from build123d import *

# Parameters (mm, degrees)
SKETCH1_W                    = 25.4
SKETCH1_H                    = 21.844
BOLT_SIZE_WIDTH_HEIGHT_DEPTH = 7.62
FRONT_CURVE_DEPTH            = 22.844
SKETCH3_W                    = 25.4
SKETCH3_H                    = 21.844
REAR_CAP_DEPTH               = 1.27
WINGS_DEPTH                  = 21.844
HOOK_DEPTH_DEPTH             = 5.08
HOOK_HEIGHT_DEPTH            = 3.81
NUT_FLANGE_CLEARANCE_R       = 1.27
DECORATION_SIZE              = 2.54
CUT_EXTRUDE1_DEPTH           = 27.9240001


with BuildPart() as part:
    # Sketch1 → Bolt Size, Width, &Height (new body)
    with BuildSketch(Plane.XY):
        Rectangle(SKETCH1_W, SKETCH1_H)
        Polygon((0, 5.842), (-5.059320409, 2.921), (-5.059320409, -2.921), (0, -5.842), (5.059320409, -2.921), (5.059320409, 2.921), align=None, mode=Mode.SUBTRACT)
    extrude(amount=BOLT_SIZE_WIDTH_HEIGHT_DEPTH)

    # Sketch2 → Front Curve (cut, through all)
    with BuildSketch(Plane(origin=(0, 10.922, 0), x_dir=(1, 0, 0), z_dir=(0, 1, 0))):
        with BuildLine():
            Line((12.7, -7.62), (12.7, -3.81))
            ThreePointArc((12.7, -3.81), (0, -4.668549118), (-12.7, -3.81))
            Line((-12.7, -3.81), (-12.7, -7.62))
            Line((-12.7, -7.62), (12.7, -7.62))
        make_face()
    extrude(amount=-FRONT_CURVE_DEPTH, mode=Mode.SUBTRACT)

    # Sketch3 → Rear Cap (add)
    with BuildSketch(Plane(origin=(0, 0, 0), x_dir=(-1, 0, 0), z_dir=(0, 0, -1))):
        Rectangle(SKETCH3_W, SKETCH3_H)
        Polygon((-3.789320409, 2.187765158), (-3.789320409, -2.187765158), (0, -4.375530316), (3.789320409, -2.187765158), (3.789320409, 2.187765158), (0, 4.375530316), align=None, mode=Mode.SUBTRACT)
    extrude(amount=REAR_CAP_DEPTH)

    # Sketch6 → Wings (add)
    with BuildSketch(Plane.XZ.offset(10.922)):
        with BuildLine():
            ThreePointArc((-12.7, 3.81), (-26.59057897, 0.844499757), (-39.878681796, -4.17234179))
            Line((-39.878681796, -4.17234179), (-37.752420533, -8.732123784))
            ThreePointArc((-37.752420533, -8.732123784), (-25.500637389, -4.079733878), (-12.7, -1.27))
            Line((-12.7, -1.27), (-12.7, 3.81))
        make_face()
        with BuildLine():
            ThreePointArc((39.878681796, -4.17234179), (26.59057897, 0.844499757), (12.7, 3.81))
            Line((12.7, 3.81), (12.7, -1.27))
            ThreePointArc((12.7, -1.27), (25.500637389, -4.079733878), (37.752420533, -8.732123784))
            Line((37.752420533, -8.732123784), (39.878681796, -4.17234179))
        make_face()
    extrude(amount=-WINGS_DEPTH)

    # Sketch7 → Hook Depth (add)
    with BuildSketch(Plane(origin=(0, 10.922, 0), x_dir=(1, 0, 0), z_dir=(0, 1, 0))):
        with BuildLine():
            Line((12.7, 1.27), (-12.7, 1.27))
            ThreePointArc((-12.7, 1.27), (-25.500637389, 4.079733878), (-37.752420533, 8.732123784))
            Line((-37.752420533, 8.732123784), (-42.90498238, -2.317580756))
            ThreePointArc((-42.90498238, -2.317580756), (-31.916762044, -6.681838924), (-20.495660276, -9.738989543))
            Line((-20.495660276, -9.738989543), (-19.05, -2.725598334))
            ThreePointArc((-19.05, -2.725598334), (0, -4.668549118), (19.05, -2.725598334))
            Line((19.05, -2.725598334), (20.495660276, -9.738989543))
            ThreePointArc((20.495660276, -9.738989543), (31.916762044, -6.681838924), (42.90498238, -2.317580756))
            Line((42.90498238, -2.317580756), (37.752420533, 8.732123784))
            ThreePointArc((37.752420533, 8.732123784), (25.500637389, 4.079733878), (12.7, 1.27))
        make_face()
    extrude(amount=HOOK_DEPTH_DEPTH)

    # Sketch8 → Hook Height (add)
    with BuildSketch(Plane.XZ.offset(-10.922)):
        with BuildLine():
            ThreePointArc((-20.495660276, 9.738989543), (-31.916762044, 6.681838924), (-42.90498238, 2.317580756))
            Line((-42.90498238, 2.317580756), (-41.831531995, 0.015558977))
            ThreePointArc((-41.831531995, 0.015558977), (-31.118228667, 4.270626689), (-19.982874273, 7.251289698))
            Line((-19.982874273, 7.251289698), (-20.495660276, 9.738989543))
        make_face()
        with BuildLine():
            Line((41.831531995, 0.015558977), (42.90498238, 2.317580756))
            ThreePointArc((42.90498238, 2.317580756), (31.916762044, 6.681838924), (20.495660276, 9.738989543))
            Line((20.495660276, 9.738989543), (19.982874273, 7.251289698))
            ThreePointArc((19.982874273, 7.251289698), (31.118228667, 4.270626689), (41.831531995, 0.015558977))
        make_face()
    extrude(amount=HOOK_HEIGHT_DEPTH)

    # Nut Flange Clearance
    nut_flange_clearance_edges = [part.edges().sort_by_distance(p)[0] for p in [
        (5.059320409, 0, 4.532819603),
        (2.530342979, 4.3811058, 4.634616736),
        (-2.530342979, 4.3811058, 4.634616736),
        (-5.059320409, 0, 4.532819603),
        (-2.530342979, -4.3811058, 4.634616736),
        (2.530342979, -4.3811058, 4.634616736),
    ]]
    fillet(nut_flange_clearance_edges, radius=NUT_FLANGE_CLEARANCE_R)

    # Decoration
    decoration_edges = [part.edges().sort_by_distance(p)[0] for p in [
        (-42.368257188, 7.112, 1.166569866),
        (-20.239267274, 7.112, 8.49513962),
        (42.368257188, 7.112, 1.166569866),
        (20.239267274, 7.112, 8.49513962),
    ]]
    chamfer(decoration_edges, length=DECORATION_SIZE)

    # Sketch9 → Cut-Extrude1 (cut, through all)
    with BuildSketch(Plane(origin=(0, 16.002, 0), x_dir=(1, 0, 0), z_dir=(0, 1, 0))):
        with BuildLine():
            Line((42.90498238, -2.317580756), (39.878681796, 4.17234179))
            ThreePointArc((39.878681796, 4.17234179), (0, -4.668549118), (-39.878681796, 4.17234179))
            Line((-39.878681796, 4.17234179), (-42.90498238, -2.317580756))
            ThreePointArc((-42.90498238, -2.317580756), (0, -11.82938635), (42.90498238, -2.317580756))
        make_face()
    extrude(amount=-CUT_EXTRUDE1_DEPTH, mode=Mode.SUBTRACT)


solid = part.part
Here's how the part is built. I have some questions about the finished solid (model axes, mm). A direction names the side the tool comes from. Coordinates: 2 decimals unless noted, no trailing zeros. Loops run counter-clockwise (first coordinate to the right, second up) from the corner with the lowest first, then second, coordinate; pieces in that order, holes last. Notation, with made-up numbers: (-39, -13.5) -> (6, -13.5) arc R15 cw to (6, 2.5) -> close; hole circle Ø1 at (48, 38.25). An arc over 180 degrees is marked (long way). Use one line per item in the form item = value. Start each with the question number.
(1) Will these pins go through, and if not, where does the flat tip stop? pin 1 (3 mm diameter, centred on x = -6.5, y = -7, fed in from +Z); pin 2 (12.5 mm diameter, centred on x = -5, y = 5, fed in from -Z); pin 3 (8 mm diameter, centred on x = 1.5, y = -2, fed in from +Z).
(2) If we section it at B-B (y = 13): Please give me the cut outline in (x, z), then the cut area to 3 significant figures.
(3) We'd pull the mould along Y, two halves only. Please class faces 1 (the face through (-1, 16.002, -1)), 2 (the face through (-1, -10.922, 0)), 3 (the face through (-2.5, 4.4, 1.7)), 4 (the face through (0, 5, -1.27)): pulls with the +Y half, pulls with the -Y half, needs draft (parallel to the pull), parting line crosses it, or undercut.
(4) On a 3-axis mill with a long thin cutter (end or side, diameter ignored), from which of +Z, -Z, +X, -X, +Y, -Y can I reach the whole of each face in a straight line? I mean faces 5 (the face through (1, -4, 0)), 6 (the face through (25.677, 2.352, -4.132)), 7 (the face through (1.921, -3.266, -0.626)). Say none if no direction works.
(5) If we section it at C-C (z = 1.5): Please give me the cut outline in (x, y), then the cut area to 3 significant figures.
(6) Please list where these lines run through material, in increasing order: line 1 along Z through (x, y) = (18, -7.25); line 2 along Z through (x, y) = (11, 14.5).
(7) If we section it at A-A (z = -6.5): Please give me the cut outline in (x, y), then the cut area to 3 significant figures.
(8) If we section it at D-D (y = 0.75): Please give me the cut outline in (x, z).
Verdict:
q1.pin_1 = 4.54
q1.pin_2 = -1.27
q1.pin_3 = 4.64
q2.outline = (-39.88, -4.17) -> (-37.75, -8.73) arc R89.33 cw to (-12.7, -1.27) -> (12.7, -1.27) arc R89.33 cw to (37.75, -8.73) -> (39.88, -4.17) arc R94.36 ccw to start
q2.area = 419 mm²
q3.face_1 = pulls with the +Y half
q3.face_2 = pulls with the -Y half
q3.face_3 = undercut
q3.face_4 = needs draft
q4.face_5 = +Z
q4.face_6 = -Z, +Y, -Y
q4.face_7 = +Z, -Z
q5.outline = (-24.25, -10.92) -> (24.25, -10.92) -> (24.25, 16) -> (-24.25, 16) -> close; hole (-5.06, -2.92) -> (0, -5.84) -> (5.06, -2.92) -> (5.06, 2.92) -> (0, 5.84) -> (-5.06, 2.92) -> close
q5.area = 1,220 mm²
q6.line_1 = -2.19 to 2.94
q6.line_2 = -1.27 to 4.03
q7.outline = (-38.79, -10.92) -> (-32.54, -10.92) -> (-32.54, 16) -> (-38.79, 16) -> close; (32.54, -10.92) -> (38.79, -10.92) -> (38.79, 16) -> (32.54, 16) -> close
q7.area = 337 mm²
q8.outline = (-39.88, -4.17) -> (-37.75, -8.73) arc R89.33 cw to (-12.7, -1.27) -> (-3.79, -1.27) -> (-3.79, 0) -> (-5.06, 0) -> (-5.06, 3.18) arc R1.27 ccw to (-6.42, 4.45) arc R94.36 ccw to start; (3.79, -1.27) -> (12.7, -1.27) arc R89.33 cw to (37.75, -8.73) -> (39.88, -4.17) arc R94.36 ccw to (6.42, 4.45) arc R1.27 ccw to (5.06, 3.18) -> (5.06, 0) -> (3.79, 0) -> close
